Geometry check sheet. Reference: the model listing, model coordinates, mm. Face numbers are marked on the shaded views. A direction names the side the tool comes from. Give positions to 0.01 mm unless a question says otherwise; leave off trailing zeros. Write each loop counter-clockwise with the first axis right and the second up, starting at its lowest first coordinate (ties: lowest second). Pieces come first, ordered by that corner, then holes. Notation, with made-up numbers: (74, -25) - (126, -25) arc R27 cw to (126, 8) - close; hole circle Ø5 at (-29.75, 10.25). An arc over 180 degrees is marked (long way). One line per question, with ' | ' between items. Start each with the question number.
Q1. Section check A-A on z = 0. Record the boundary of the cut face in (x, y), and give its area (3 significant figures).
Q2. Set-up check for the marked faces 1, 2 and 3: record each of +Z, -Z, +X, -X, +Y, -Y from which the full face is reachable in a straight line by a thin tool's end or side.
Q3. Gauge pin test, flat ends, axial feed: P1, Ø1.7, axis at x = -8.5, z = -1, coming from the -Y side; P2, Ø18, axis at y = 39, z = 7.5, coming from the -X side; P3, Ø2, axis at y = 21, z = 12, coming from the -X side. Record the tip position at first contact, or that the pin passes through.
Q4. Section check D-D on z = -8.5. Record the boundary of the cut face in (x, y), and give its area (3 significant figures).
Q5. Release check for a two-part mould opening along Z. For the marked faces 4, 5 and 6 record: +Z half, -Z half, draft (parallel to the pull), parting line (faces both ways), or undercut.
Q6. Section check B-B on y = 12.7. Record the boundary of the cut face in (x, z).
Q7. Section check C-C on z = 12.7. Count the separate pieces of the cut face and the enclosed holes in it, and give its area (3 significant figures).
Q8. Thickness scan on L1, parallel to Z at x = -3.5, y = 12.7; L2, parallel to Z at x = -5, y = 25.4; L3, parallel to Y at x = -2.2, z = 0. Record the ranges inside material, lowest first. Write a range as [from, to].
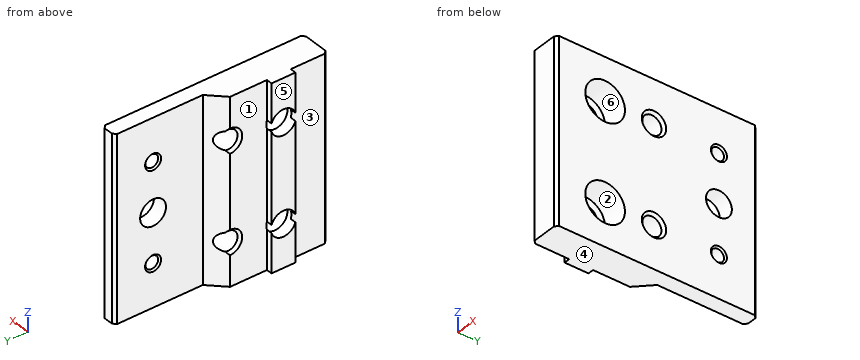
Autodesk Inventor part; units mm, degrees
ref_plane "to_pad1_XY" through (-3.9624, 42.291, -12.7) normal (1, 0, 0) x (0, 0, -1)
ref_plane "to_pad1_YZ" through (-3.9624, 42.291, -12.7) normal (0, 0, -1) x (0, 1, 0)
ref_plane "to_pad1_ZX" through (-3.9624, 42.291, -12.7) normal (0, 1, 0) x (1, 0, 0)
sketch "Sketch_1" plane through (0, 0, 0) normal (0, 0, 1) x (1, 0, 0)
  line L0 (-9.4488, 15.7988) -> (-9.4488, 9.6012)
  line L1 (-9.4488, 9.6012) -> (-7.9248, 9.6012)
  line L2 (-7.9248, 9.6012) -> (-7.9248, 0.762)
  line L3 (-7.9248, 0.762) -> (-7.1628, 0)
  line L4 (-7.1628, 0) -> (-0.762, 0)
  line L5 (-0.762, 0) -> (0, 0.762)
  line L6 (0, 0.762) -> (0, 51.6128)
  line L7 (0, 51.6128) -> (-0.762, 52.3748)
  line L8 (-0.762, 52.3748) -> (-3.2004, 52.3748)
  line L9 (-3.2004, 52.3748) -> (-3.9624, 51.6128)
  line L10 (-3.9624, 51.6128) -> (-3.9624, 29.3624)
  line L11 (-3.9624, 29.3624) -> (-7.9248, 25.4)
  line L12 (-7.9248, 25.4) -> (-7.9248, 15.7988)
  line L13 (-7.9248, 15.7988) -> (-9.4488, 15.7988)
extrude "Extrusion1" add sketch "Sketch_1" along normal mid plane 47.625
sketch "Sketch_2" plane through (0, 0, 12.7) normal (0, 0, 1) x (1, 0, 0)
  line L0 (0, 42.291) -> (-3.9624, 42.291)
  line L1 (-3.9624, 42.291) -> (-3.9624, 44.3738)
  line L2 (-3.9624, 44.3738) -> (-3.5331, 43.9445)
  line L3 (-3.5331, 43.9445) -> (-0.4293, 43.9445)
  line L4 (-0.4293, 43.9445) -> (0, 44.3738)
  line L5 (0, 44.3738) -> (0, 42.291)
  line L6 (0, 42.291) -> (-3.9624, 42.291)
revolve "Revolution1" cut sketch "Sketch_2" angle 360 about axis through (0, 42.291, 12.7) along (1, 0, 0)
thread "Thread1"
pattern_linear "Rectangular Pattern1" count 2 spacing 25.4 along (0, 0, -1) of "Revolution1"
sketch "Sketch_4" plane through (0, 0, 12.7) normal (0, 0, 1) x (1, 0, 0)
  line L0 (0, 25.4) -> (-7.9248, 25.4)
  line L1 (-7.9248, 25.4) -> (-7.9248, 28.575)
  line L2 (-7.9248, 28.575) -> (-7.2377, 27.8879)
  line L3 (-7.2377, 27.8879) -> (-0.6871, 27.8879)
  line L4 (-0.6871, 27.8879) -> (0, 28.575)
  line L5 (0, 28.575) -> (0, 25.4)
  line L6 (0, 25.4) -> (-7.9248, 25.4)
revolve "Revolution2" cut sketch "Sketch_4" angle 360 about axis through (0, 25.4, 12.7) along (1, 0, 0)
thread "Thread2"
pattern_linear "Rectangular Pattern2" count 2 spacing 25.4 along (0, 0, -1) of "Revolution2"
sketch "Sketch4" plane through (0, 0.762, 23.8125) normal (1, 0, 0) x (0, 0, -1)
  point P0 (11.1125, 11.938)
hole "Hole1" at (0, 12.7, 12.7) direction (-1, 0, 0) diameter 6.5278 depth 9.4488 counterbore diameter 10.3124 counterbore depth 6.604
pattern_linear "Rectangular Pattern3" count 2 spacing 25.4 along (0, 0, -1) of "Hole1"
sketch "Sketch5" plane through (0, 0.762, 23.8125) normal (1, 0, 0) x (0, 0, -1)
  point P0 (23.8125, 41.529)
hole "Hole2" at (0, 42.291, 0) direction (-1, 0, 0) diameter 6.731 depth 3.9624
ref_plane "to_pad1_XY" through (-3.9624, 42.291, -12.7) normal (1, 0, 0) x (0, 0, -1)
ref_plane "to_pad1_YZ" through (-3.9624, 42.291, -12.7) normal (0, 0, -1) x (0, 1, 0)
ref_plane "to_pad1_ZX" through (-3.9624, 42.291, -12.7) normal (0, 1, 0) x (1, 0, 0)
ref_plane "to_pad2_XY" through (-3.9624, 42.291, -12.7) normal (1, 0, 0) x (0, 0, -1)
ref_plane "to_pad2_YZ" through (-3.9624, 42.291, -12.7) normal (0, 0, -1) x (0, 1, 0)
ref_plane "to_pad2_ZX" through (-3.9624, 42.291, -12.7) normal (0, 1, 0) x (1, 0, 0)
ref_plane "to_profile_XY" through (-7.9248, 12.7, 0) normal (1, 0, 0) x (0, 0, -1)
ref_plane "to_profile_YZ" through (-7.9248, 12.7, 0) normal (0, 0, -1) x (0, 1, 0)
ref_plane "to_profile_ZX" through (-7.9248, 12.7, 0) normal (0, 1, 0) x (1, 0, 0)
ref_plane "to_screw_1_XY" through (-6.604, 12.7, 12.7) normal (1, 0, 0) x (0, 0, -1)
ref_plane "to_screw_1_YZ" through (-6.604, 12.7, 12.7) normal (0, 0, -1) x (0, 1, 0)
ref_plane "to_screw_1_ZX" through (-6.604, 12.7, 12.7) normal (0, 1, 0) x (1, 0, 0)
ref_plane "to_screw_2_XY" through (-6.604, 12.7, -12.7) normal (1, 0, 0) x (0, 0, -1)
ref_plane "to_screw_2_YZ" through (-6.604, 12.7, -12.7) normal (0, 0, -1) x (0, 1, 0)
ref_plane "to_screw_2_ZX" through (-6.604, 12.7, -12.7) normal (0, 1, 0) x (1, 0, 0)
ref_plane "to_screw_3_XY" through (-6.604, 12.7, -12.7) normal (1, 0, 0) x (0, 0, -1)
ref_plane "to_screw_3_YZ" through (-6.604, 12.7, -12.7) normal (0, 0, -1) x (0, 1, 0)
ref_plane "to_screw_3_ZX" through (-6.604, 12.7, -12.7) normal (0, 1, 0) x (1, 0, 0)
ref_plane "to_screw_4_XY" through (-6.604, 12.7, -12.7) normal (1, 0, 0) x (0, 0, -1)
ref_plane "to_screw_4_YZ" through (-6.604, 12.7, -12.7) normal (0, 0, -1) x (0, 1, 0)
ref_plane "to_screw_4_ZX" through (-6.604, 12.7, -12.7) normal (0, 1, 0) x (1, 0, 0)
properties part number "6760_p"
Working result:
1) outline: (-9.45, 9.6) - (-7.92, 9.6) - (-7.92, 0.76) - (-7.16, 0) - (-0.76, 0) - (0, 0.76) - (0, 38.93) - (-3.96, 38.93) - (-3.96, 29.36) - (-7.92, 25.4) - (-7.92, 15.8) - (-9.45, 15.8) - close; (-3.96, 45.66) - (0, 45.66) - (0, 51.61) - (-0.76, 52.37) - (-3.2, 52.37) - (-3.96, 51.61) - close | area: 298 mm2
2) face 1: +Z, -Z, -X, +Y | face 2: +X | face 3: +Z, -Z, -X, -Y
3) P1: stops at y = 0.49 | P2: stops at x = -3.96 | P3: stops at x = -7.92
4) outline: (-9.45, 9.6) - (-7.92, 9.6) - (-7.92, 0.76) - (-7.16, 0) - (-0.76, 0) - (0, 0.76) - (0, 9.71) - (-6.6, 9.71) - (-6.6, 15.69) - (0, 15.69) - (0, 51.61) - (-0.76, 52.37) - (-3.2, 52.37) - (-3.96, 51.61) - (-3.96, 29.36) - (-7.92, 25.4) - (-7.92, 15.8) - (-9.45, 15.8) - close | area: 285 mm2
5) face 4: -Z half | face 5: draft | face 6: undercut
6) outline: (-9.45, -23.81) - (0, -23.81) - (0, -17.86) - (-6.6, -17.86) - (-6.6, -15.96) - (-9.45, -15.96) - close; (-9.45, -9.44) - (-6.6, -9.44) - (-6.6, -7.54) - (0, -7.54) - (0, 7.54) - (-6.6, 7.54) - (-6.6, 9.44) - (-9.45, 9.44) - close; (-9.45, 15.96) - (-6.6, 15.96) - (-6.6, 17.86) - (0, 17.86) - (0, 23.81) - (-9.45, 23.81) - close
7) separate pieces: 4 | enclosed holes: 0 | area: 188 mm2
8) L1: z = [-23.81, -17.86], [-7.54, 7.54], [17.86, 23.81] | L2: z = [-23.81, -15.19], [-10.21, 10.21], [15.19, 23.81] | L3: y = [0, 38.93], [45.66, 52.37]
